Input: part model. Units: mm. Frame: model coordinates. A direction names the side the tool comes from. Coordinates: 2 decimals unless noted, no trailing zeros. Write each loop counter-clockwise with the first axis right and the second up, starting at its lowest first coordinate (ties: lowest second). Pieces come first, ordered by that corner, then holes. Notation, with made-up numbers: M -14,-9 L 20,-9 A8 ccw 20,4 Z; hole C -2.5,-24.5 d5. An arc over 180 degrees is marked long. Use CSV: the item, a comma, the result in double quotes.
```python
from build123d import *

# Parameters (mm, degrees)
SKETCH1_W           = 20
SKETCH1_H           = 2
BOSS_EXTRUDE1_DEPTH = 1
SKETCH2_R           = 0.35
BOSS_EXTRUDE3_DEPTH = 2.5
CHAMFER2_SIZE       = 0.3
CHAMFER4_SIZE       = 0.3
CHAMFER5_SIZE       = 0.3
SKETCH4_W           = 4.351090726
SKETCH4_H           = 1.4
BOSS_EXTRUDE4_DEPTH = 0.75


with BuildPart() as part:
    # Sketch1 → Boss-Extrude1 (new body)
    with BuildSketch(Plane.XY):
        Rectangle(SKETCH1_W, SKETCH1_H)
    extrude(amount=BOSS_EXTRUDE1_DEPTH)

    # Sketch2 → Boss-Extrude3 (add)
    with BuildSketch(Plane.XY.offset(1)):
        with Locations((-7.5, 0)):
            Circle(SKETCH2_R)
    extrude(amount=BOSS_EXTRUDE3_DEPTH)

    # Chamfer2
    chamfer2_edges = [part.edges().sort_by_distance(p)[0] for p in [
        (10, 1, 0.5),
    ]]
    chamfer(chamfer2_edges, length=CHAMFER2_SIZE)

    # Chamfer4
    # the kernel refuses this chamfer: 0.3 mm, written as the material it takes off along each edge
    with BuildSketch(Plane(origin=(10, 1.471504896, 0), x_dir=(-0.9996219169112968, 0, -0.02749587661058633), z_dir=(0, -1, 0))) as chamfer4_piece_1:
        Polygon((CHAMFER4_SIZE * 0.999621916911, -CHAMFER4_SIZE * 0.0274958766106), (-CHAMFER4_SIZE * 0.0274958766106, -CHAMFER4_SIZE * 0.999621916911), (0, 0), align=None)
    extrude(amount=3.243009793, mode=Mode.SUBTRACT)
    with BuildSketch(Plane(origin=(10, 1.471504896, 1), x_dir=(-0.9996219169112968, 0, 0.027495876610586622), z_dir=(0, -1, 0))) as chamfer4_piece_2:
        Polygon((CHAMFER4_SIZE * 0.999621916911, CHAMFER4_SIZE * 0.0274958766106), (-CHAMFER4_SIZE * 0.0274958766106, CHAMFER4_SIZE * 0.999621916911), (0, 0), align=None)
    extrude(amount=3.243009793, mode=Mode.SUBTRACT)
    with BuildSketch(Plane(origin=(10.771504896, -1, 1), x_dir=(0, 0.9996219169112968, 0.027495876610586632), z_dir=(-1, 0, 0))) as chamfer4_piece_3:
        Polygon((CHAMFER4_SIZE * 0.999621916911, CHAMFER4_SIZE * 0.0274958766106), (-CHAMFER4_SIZE * 0.0274958766106, CHAMFER4_SIZE * 0.999621916911), (0, 0), align=None)
    extrude(amount=21.543009793, mode=Mode.SUBTRACT)
    with BuildSketch(Plane(origin=(-10.771504896, 1, 0), x_dir=(0, 0.027495876610586632, 0.9996219169112968), z_dir=(1, 0, 0))) as chamfer4_piece_4:
        Polygon((CHAMFER4_SIZE * 0.999621916911, CHAMFER4_SIZE * 0.0274958766106), (-CHAMFER4_SIZE * 0.0274958766106, CHAMFER4_SIZE * 0.999621916911), (0, 0), align=None)
    extrude(amount=21.243009793, mode=Mode.SUBTRACT)
    with BuildSketch(Plane(origin=(-10.771504896, 1, 1), x_dir=(0, 0.027495876610586632, -0.9996219169112968), z_dir=(1, 0, 0))) as chamfer4_piece_5:
        Polygon((CHAMFER4_SIZE * 0.999621916911, -CHAMFER4_SIZE * 0.0274958766106), (-CHAMFER4_SIZE * 0.0274958766106, -CHAMFER4_SIZE * 0.999621916911), (0, 0), align=None)
    extrude(amount=21.243009793, mode=Mode.SUBTRACT)

    # Chamfer5
    chamfer5_edges = [part.edges().sort_by_distance(p)[0] for p in [
        (-10, 0, 1),
        (-10, -0.15, 0),
        (-0.15, -1, 0),
    ]]
    chamfer(chamfer5_edges, length=CHAMFER5_SIZE)

    # Sketch4 → Boss-Extrude4 (add)
    with BuildSketch(Plane(origin=(0, 0, 0), x_dir=(-1, 0, 0), z_dir=(0, 0, -1))):
        with Locations((7.524454637, 0)):
            Rectangle(SKETCH4_W, SKETCH4_H)
    extrude(amount=BOSS_EXTRUDE4_DEPTH)


solid = part.part
```
1. Section C-C (x = -7.5). Return loops of the section in (y, z).
Resolved:
outline,"M -1,0.3 L -0.7,0 L -0.7,-0.75 L 0.7,-0.75 L 0.7,0 L 1,0.3 L 1,0.7 L 0.7,1 L 0.35,1 L 0.35,3.5 L -0.35,3.5 L -0.35,1 L -0.7,1 L -1,0.7 Z"
2. Section D-D (z = -0.25). Return loops of the section in (x, y), then the cut area to 3 significant figures.
Resolved:
outline,"M -9.7,-0.7 L -5.35,-0.7 L -5.35,0.7 L -9.7,0.7 Z"
area,"6.09 mm^2"
3. Section A-A (x = -3). Return loops of the section in (y, z).
Resolved:
outline,"M -1,0.3 L -0.7,0 L 0.7,0 L 1,0.3 L 1,0.7 L 0.7,1 L -0.7,1 L -1,0.7 Z"
4. Contact query for flat-ended pins moving along their axis: pin 1 Ø0.8 at (y, z) = (-0.5, -0.5) entering from +X; pin 2 Ø0.7 at (x, y) = (-4.5, 0) entering from +Z; pin 3 Ø0.6 at (y, z) = (0, -0.5) entering from -X. Output: stop coordinate, or through.
Resolved:
pin 1,"stops at x = -5.35"
pin 2,"stops at z = 1"
pin 3,"stops at x = -9.7"
5. Section B-B (y = 0). Return loops of the section in (x, z), then the cut area to 3 significant figures.
Resolved:
outline,"M -10,0.3 L -9.7,0 L -9.7,-0.75 L -5.35,-0.75 L -5.35,0 L 9.7,0 L 10,0.3 L 10,0.7 L 9.7,1 L -7.15,1 L -7.15,3.5 L -7.85,3.5 L -7.85,1 L -9.7,1 L -10,0.7 Z"
area,"24.8 mm^2"
6. Material intervals for line 1 (X direction, y = 0.05, z = -0.1); line 2 (Z direction, x = -6, y = 0.25); line 3 (Z direction, x = 7.5, y = -0.4), sorted ascending. Write a range as [from, to].
Resolved:
line 1,"x = [-9.7, -5.35]"
line 2,"z = [-0.75, 1]"
line 3,"z = [0, 1]"
7. Access query for faces 1 (the flat face through (-7, 0, -0.75)), 2 (the flat face through (2, 0, 0)). Directions: +Z, -Z, +X, -X, +Y, -Y. A direction counts if a zero-diameter tool reaches every point of the face in a straight line with its end or side. Return the directions, or none.
Resolved:
face 1,"-Z, +X, -X, +Y, -Y"
face 2,"-Z, +X, +Y, -Y"
